Could you check a few things on this model? Use its own coordinates, in mm. A direction names the side the tool comes from. Coordinates: 2 decimals unless noted, no trailing zeros. Write each loop counter-clockwise with the first axis right and the second up, starting at its lowest first coordinate (ties: lowest second). Pieces come first, ordered by that corner, then holes.
Item 1: For P1, Ø1, axis at x = 2, z = 3.5, coming from the -Y side; P2, Ø1.5, axis at y = 2, z = 1.5, coming from the -X side; P3, Ø3, axis at x = 2, y = -2, coming from the +Z side; P4, Ø3, axis at x = -1.5, z = 6, coming from the +Y side, each with a flat end and sliding along its axis, tell me the tip position at first contact or that it passes through.
Item 2: I want a section at C-C on z = 1. Please give me the cut outline in (x, y) (3 decimals).
Item 3: I want a section at D-D on z = 6. Please give me the cut outline in (x, y), then the cut area to 3 significant figures.
Item 4: I want a section at A-A on y = 0. Please give me the cut outline in (x, z) (3 decimals).
Item 5: If I drill on probe 1 along Z at (x, y) = (0, 2); probe 2 along X at (y, z) = (-0.5, 1.5); probe 3 along X at (y, z) = (0.75, 3.5), over which ranges is the centre line in solid material (lowest first)?
Item 6: Which directions (+Z, -Z, +X, -X, +Y, -Y) give clear straight access to the entire face, cutting with the end or side of a thin tool? Please do faces 1 (the cylindrical face through (0.65, 1.01, 4.43)), 2 (the flat face through (0, 0, 0)).
from build123d import *

# Parameters (mm, degrees)
SKETCH_R     = 3.175
PAD_DEPTH    = 2.7
SKETCH001_R  = 1.2
PAD001_DEPTH = 4
CHAMFER_SIZE = 0.5


with BuildPart() as part:
    # Sketch → Pad (new body)
    with BuildSketch(Plane.XY):
        Circle(SKETCH_R)
    extrude(amount=PAD_DEPTH)

    # Sketch001 → Pad001 (new body)
    with BuildSketch(Plane.XY.offset(2.7)):
        Circle(SKETCH001_R)
    extrude(amount=PAD001_DEPTH)

    # Chamfer
    chamfer_edges = [part.edges().sort_by_distance(p)[0] for p in [
        (-1.2, 0, 6.7),
    ]]
    chamfer(chamfer_edges, length=CHAMFER_SIZE)


solid = part.part
Response values:
1. P1: passes through
1. P2: stops at x = -2.92
1. P3: stops at z = 2.7
1. P4: stops at y = 1.2
2. outline: circle Ø6.35 at (0, 0)
3. outline: circle Ø2.4 at (0, 0)
3. area: 4.52 mm2
4. outline: (-3.175, 0) - (3.175, 0) - (3.175, 2.7) - (1.2, 2.7) - (1.2, 6.2) - (0.7, 6.7) - (-0.7, 6.7) - (-1.2, 6.2) - (-1.2, 2.7) - (-3.175, 2.7) - close
5. probe 1: z = 0 to 2.7
5. probe 2: x = -3.14 to 3.14
5. probe 3: x = -0.94 to 0.94
6. face 1: +Z
6. face 2: -Z, +X, -X, +Y, -Y
